CAD build for the part. Positions are in the model's coordinates, mm. A direction names the side the tool comes from. Coordinates: 2 decimals unless noted, no trailing zeros. Loops run counter-clockwise (first coordinate to the right, second up) from the corner with the lowest first, then second, coordinate; pieces in that order, holes last. Notation, with made-up numbers: (-39, 75.5) -> (-1, 75.5) arc R11 cw to (-1, 92.5) -> close; hole circle Ø5 at (15, 60). An arc over 180 degrees is marked (long way). Write each question's results on one line, items separated by ' | '.
from build123d import *

# Parameters (mm, degrees)
SKETCH1_W           = 62.755543402
SKETCH1_H           = 8.222921835
BOSS_EXTRUDE1_DEPTH = 10
SKETCH1_3_R         = 2.55
SKETCH1_3_W         = 2.689412068
SKETCH1_3_H         = 4.439494762
CUT_EXTRUDE1_DEPTH  = 10
SKETCH1_4_R         = 2.8
SKETCH1_4_R_2       = 2.775
SKETCH1_4_R_3       = 2.75
SKETCH1_4_R_4       = 2.725
SKETCH1_4_R_5       = 2.825
SKETCH1_4_R_6       = 2.85
SKETCH1_4_R_7       = 2.875
SKETCH1_4_R_8       = 2.9
CUT_EXTRUDE2_DEPTH  = 1.2


with BuildPart() as part:
    # Sketch1 → Boss-Extrude1 (new body)
    with BuildSketch(Plane.XY):
        with Locations((31.377771701, 4.111460918)):
            Rectangle(SKETCH1_W, SKETCH1_H)
    extrude(amount=BOSS_EXTRUDE1_DEPTH)

    # Sketch1<3> → Cut-Extrude1 (cut)
    with BuildSketch(Plane.XY):
        with Locations((8.746479161, 4.111460918)):
            Circle(SKETCH1_3_R)
        with Locations((16.214765516, 4.111460918)):
            Circle(SKETCH1_3_R)
        with Locations((23.139004522, 4.111460918)):
            Circle(SKETCH1_3_R)
        with Locations((30.557832028, 4.111460918)):
            Circle(SKETCH1_3_R)
        with Locations((37.630447583, 4.111460918)):
            Circle(SKETCH1_3_R)
        with Locations((44.752521989, 4.111460918)):
            Circle(SKETCH1_3_R)
        with Locations((51.627302144, 4.111460918)):
            Circle(SKETCH1_3_R)
        with Locations((58.650458849, 4.111460918)):
            Circle(SKETCH1_3_R)
        with Locations((3.166946189, 4.661409139)):
            Rectangle(SKETCH1_3_W, SKETCH1_3_H)
    extrude(amount=CUT_EXTRUDE1_DEPTH, mode=Mode.SUBTRACT)

    # Sketch1<4> → Cut-Extrude2 (cut)
    with BuildSketch(Plane.XY):
        with Locations((8.746479161, 4.111460918)):
            Circle(SKETCH1_4_R)
        with Locations((16.214765516, 4.111460918)):
            Circle(SKETCH1_4_R_2)
        with Locations((23.139004522, 4.111460918)):
            Circle(SKETCH1_4_R_3)
        with Locations((30.557832028, 4.111460918)):
            Circle(SKETCH1_4_R_4)
        with Locations((37.630447583, 4.111460918)):
            Circle(SKETCH1_4_R_5)
        with Locations((44.752521989, 4.111460918)):
            Circle(SKETCH1_4_R_6)
        with Locations((51.627302144, 4.111460918)):
            Circle(SKETCH1_4_R_7)
        with Locations((58.650458849, 4.111460918)):
            Circle(SKETCH1_4_R_8)
    extrude(amount=CUT_EXTRUDE2_DEPTH, mode=Mode.SUBTRACT)


solid = part.part
1) Drill centre lines: L1, parallel to Y at x = 45, z = 4.75; L2, parallel to Y at x = 37.5, z = 2.5; L3, parallel to Z at x = 53.5, y = 6. Where is each one in solid material? Low to high. Write a range as from..to.
Outcome:
L1: y = 0..1.57, 6.65..8.22 | L2: y = 0..1.56, 6.66..8.22 | L3: z = 1.2..10
2) Pin check, flat tip, straight feed: pin 1 (3 mm diameter, centred on x = 50.5, y = 5, fed in from -Z). Stop position of the tip, or through.
Outcome:
pin 1: stops at z = 0
3) Which spindle directions (+Z, -Z, +X, -X, +Y, -Y) get a long thin tool onto all of the face, cutting with end or side? Do faces 3 (the cylindrical face through (49.346, 2.362, 0.592)), 4 (the flat face through (3, 2.442, 5)). Say none if no direction does.
Outcome:
face 3: -Z | face 4: +Z, -Z
4) Slice it at A-A (x = 45.5). Write the cut outline in (y, z).
Outcome:
outline: (0, 0) -> (1.36, 0) -> (1.36, 1.2) -> (1.67, 1.2) -> (1.67, 10) -> (0, 10) -> close; (6.55, 1.2) -> (6.86, 1.2) -> (6.86, 0) -> (8.22, 0) -> (8.22, 10) -> (6.55, 10) -> close
5) Two-plate mould, pull along X, no slides. Class faces 1 (the flat face through (62.756, 4, 5)), 2 (the cylindrical face through (61.417, 4.983, 0.592)): pulls with the +X half, pulls with the -X half, needs draft (parallel to the pull), parting line crosses it, or undercut.
Outcome:
face 1: pulls with the +X half | face 2: undercut
6) Slice it at B-B (z = 6.75). Count the separate pieces of the cut face and the enclosed holes in it, then the cut area to 3 significant figures.
Outcome:
separate pieces: 1 | enclosed holes: 9 | area: 341 mm^2
7) Slice it at D-D (x = 53). Write the cut outline in (y, z), then the cut area to 3 significant figures.
Outcome:
outline: (0, 0) -> (1.59, 0) -> (1.59, 1.2) -> (1.96, 1.2) -> (1.96, 10) -> (0, 10) -> close; (6.26, 1.2) -> (6.64, 1.2) -> (6.64, 0) -> (8.22, 0) -> (8.22, 10) -> (6.26, 10) -> close | area: 38.3 mm^2
